Answer from the drawing. Dimensions are ordinates in mm from the lowest x, y and z of the part. Give positions to 0.01 mm unless a question says otherwise; leave off trailing zeros. Loops run counter-clockwise (first coordinate to the right, second up) from the corner with the lowest first, then second, coordinate; pieces in that order, holes last.
Item 1: Section A-A, the plane z = 4.25 is taken. Give the number of separate pieces and of enclosed holes in the cut face, and give its area (3 significant figures).
Item 2: Section B-B, the plane y = 9.75 is taken. Give the vertices of the cut face in (x, z).
Item 3: Consider line 1 along X through (y, z) = (12.5, 9.5); line 2 along Y through (x, z) = (12.5, 3.5); line 3 along X through (y, z) = (10.75, 6.5). Determine where each line is inside the solid, lowest interval first.
Item 4: Each of these flat-tipped pins is pushed along its axis until it touches: pin 1 Ø10 at (x, y) = (12.5, 12.5) entering from +Z; pin 2 Ø2 at (y, z) = (10, 8.5) entering from -X; pin 3 Ø4 at (y, z) = (21, 5.5) entering from +X; pin 4 Ø6 at (y, z) = (18.5, 3) entering from -X. Where does it stop, or does it pass through?
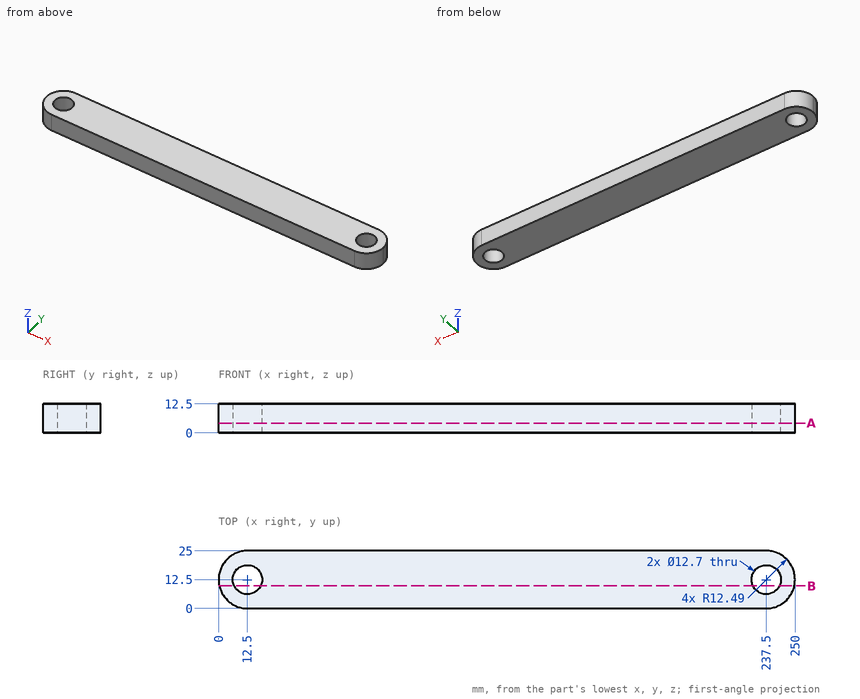
Worked answers:
1. separate pieces: 1
1. enclosed holes: 2
1. area: 5,860 mm2
2. outline: (0.3, 0) - (6.78, 0) - (6.78, 12.5) - (0.3, 12.5) - close; (18.22, 0) - (231.78, 0) - (231.78, 12.5) - (18.22, 12.5) - close; (243.22, 0) - (249.7, 0) - (249.7, 12.5) - (243.22, 12.5) - close
3. line 1: x = 0 to 6.15, 18.85 to 231.15, 243.85 to 250
3. line 2: y = 0 to 6.15, 18.85 to 25
3. line 3: x = 0.12 to 6.4, 18.6 to 231.4, 243.6 to 249.88
4. pin 1: passes through
4. pin 2: stops at x = 0.09
4. pin 3: stops at x = 248.18
4. pin 4: stops at x = 0.36
